from build123d import *

# Parameters (mm, degrees)
SKETCH1_R           = 6.35
SKETCH1_R_2         = 4.445
BOSS_EXTRUDE4_DEPTH = 3.175
FILLET1_R           = 7.62
FILLET2_R           = 2.54


with BuildPart() as part:
    # Sketch1 → Boss-Extrude4 (new body)
    with BuildSketch(Plane(origin=(0, 0, 0), x_dir=(1, 0, 0), z_dir=(0, 1, 0))):
        with BuildLine():
            ThreePointArc((132.708902298, 34.70274992), (130.780561186, 44.591665065), (121.053534347, 47.21732518))
            Line((121.053534347, 47.21732518), (-2.940598336, 9.725146859))
            ThreePointArc((-2.940598336, 9.725146859), (-10.050698784, -1.486288652), (0, -10.16))
            Line((0, -10.16), (108.585, -10.16))
            ThreePointArc((108.585, -10.16), (114.347311535, -8.367877017), (118.076794146, -3.623733419))
            Line((118.076794146, -3.623733419), (132.708902298, 34.70274992))
        make_face()
        with BuildLine():
            Line((5.835638087, 8.316906163), (30.582028831, 15.535454115))
            Line((30.582028831, 15.535454115), (52.49530672, -6.35))
            Line((52.49530672, -6.35), (7.931147458, -6.35))
            ThreePointArc((7.931147458, -6.35), (10.057864095, 1.437000294), (5.835638087, 8.316906163))
        make_face(mode=Mode.SUBTRACT)
        Polygon((33.363906977, 16.346930867), (92.350223331, 33.55330078), (54.291359033, -4.553949138), align=None, mode=Mode.SUBTRACT)
        with BuildLine():
            Line((94.419089716, 32.030410831), (103.665421891, 8.889507929))
            ThreePointArc((103.665421891, 8.889507929), (98.617756781, 1.969685918), (100.653852542, -6.35))
            Line((100.653852542, -6.35), (56.087411343, -6.35))
            Line((56.087411343, -6.35), (94.419089716, 32.030410831))
        make_face(mode=Mode.SUBTRACT)
        with BuildLine():
            Line((96.107879032, 34.649412861), (114.478426945, 40.008120819))
            ThreePointArc((114.478426945, 40.008120819), (116.909216359, 31.534937584), (125.250600093, 28.684518542))
            Line((125.250600093, 28.684518542), (117.182643526, 5.413513258))
            ThreePointArc((117.182643526, 5.413513258), (112.325487778, 9.446393554), (106.024105012, 9.831958953))
            Line((106.024105012, 9.831958953), (96.107879032, 34.649412861))
        make_face(mode=Mode.SUBTRACT)
        with Locations(Location((108.585, 0, 0), (0, 0, 270))):
            Circle(SKETCH1_R, mode=Mode.SUBTRACT)
        with Locations(Location((123.810345287, 38.1, 0), (0, 0, 270))):
            Circle(SKETCH1_R_2, mode=Mode.SUBTRACT)
        with Locations(Location((0, 0, 0), (0, 0, 270))):
            Circle(SKETCH1_R, mode=Mode.SUBTRACT)
    extrude(amount=-BOSS_EXTRUDE4_DEPTH)

    # Fillet1
    fillet1_edges = [part.edges().sort_by_distance(p)[0] for p in [
        (5.835638087, -1.5875, -8.316906163),
        (7.931147458, -1.5875, 6.35),
        (100.653852542, -1.5875, 6.35),
        (125.250600093, -1.5875, -28.684518542),
        (114.478426945, -1.5875, -40.008120819),
        (117.182643526, -1.5875, -5.413513258),
    ]]
    fillet(fillet1_edges, radius=FILLET1_R)

    # Fillet2
    fillet2_edges = [part.edges().sort_by_distance(p)[0] for p in [
        (92.350223331, -1.5875, -33.55330078),
        (33.363906977, -1.5875, -16.346930867),
        (54.291359033, -1.5875, 4.553949138),
        (30.582028831, -1.5875, -15.535454115),
        (52.49530672, -1.5875, 6.35),
        (103.665421891, -1.5875, -8.889507929),
        (94.419089716, -1.5875, -32.030410831),
        (56.087411343, -1.5875, 6.35),
        (96.107879032, -1.5875, -34.649412861),
        (106.024105012, -1.5875, -9.831958953),
    ]]
    fillet(fillet2_edges, radius=FILLET2_R)


solid = part.part
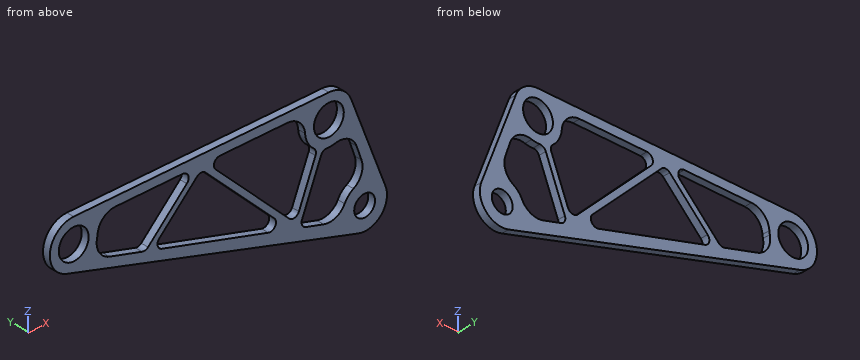
Read the model definition and answer for the solid it produces. Units are mm, in the model's axes. Coordinates: 2 decimals unless noted, no trailing zeros. Loops run counter-clockwise (first coordinate to the right, second up) from the corner with the lowest first, then second, coordinate; pieces in that order, holes last.
Q1. Each of these flat-tipped pins is pushed along its axis until it touches: pin 1 Ø12 at (x, z) = (98.5, -15.5) entering from +Y; pin 2 Ø1 at (x, y) = (63, -3) entering from -Z; pin 3 Ø1 at (y, z) = (-1.5, -7) entering from +X. Where does it stop, or does it pass through?
Q2. Consider probe 1 along Z at (x, y) = (68.5, -1.5); probe 2 along Z at (x, y) = (42, -1.8); probe 3 along X at (y, z) = (-2.3, -9). Determine where each line is inside the solid, lowest interval first.
Q3. The part is cut by section A-A on x = 74.5. Write down the section's boundary in (y, z) (3 decimals), and give its area (3 significant figures).
Q4. The part is cut by section B-B on y = -1.75. Give the number of separate pieces and of enclosed holes in the cut face, and give its area (3 significant figures).
Results below:
1. pin 1: stops at y = 0
1. pin 2: stops at z = -29.81
1. pin 3: stops at x = 122.32
2. probe 1: z = -31.33 to -26.6, -9.67 to -6.08, 6.35 to 10.16
2. probe 2: z = -23.31 to -18.87, -7.72 to -4.13, 6.35 to 10.16
2. probe 3: x = -4.71 to 11.86, 37.13 to 40.72, 67.83 to 71.42, 102.95 to 122.9
3. outline: (-3.175, -33.141) - (0, -33.141) - (0, -28.346) - (-3.175, -28.346) - close; (-3.175, -15.68) - (0, -15.68) - (0, -12.086) - (-3.175, -12.086) - close; (-3.175, 6.35) - (0, 6.35) - (0, 10.16) - (-3.175, 10.16) - close
3. area: 38.7 mm2
4. separate pieces: 1
4. enclosed holes: 7
4. area: 2,070 mm2
